The drawing under review shows one solid part. Ordinate dimensions are in mm from its lowest x, y, z. Round coordinates to 2 decimals unless told otherwise and drop trailing zeros. Order: outer loops, then holes, each group sorted by start corner. A loop starts at its lowest first (then second) coordinate and runs counter-clockwise, first axis right, second up.
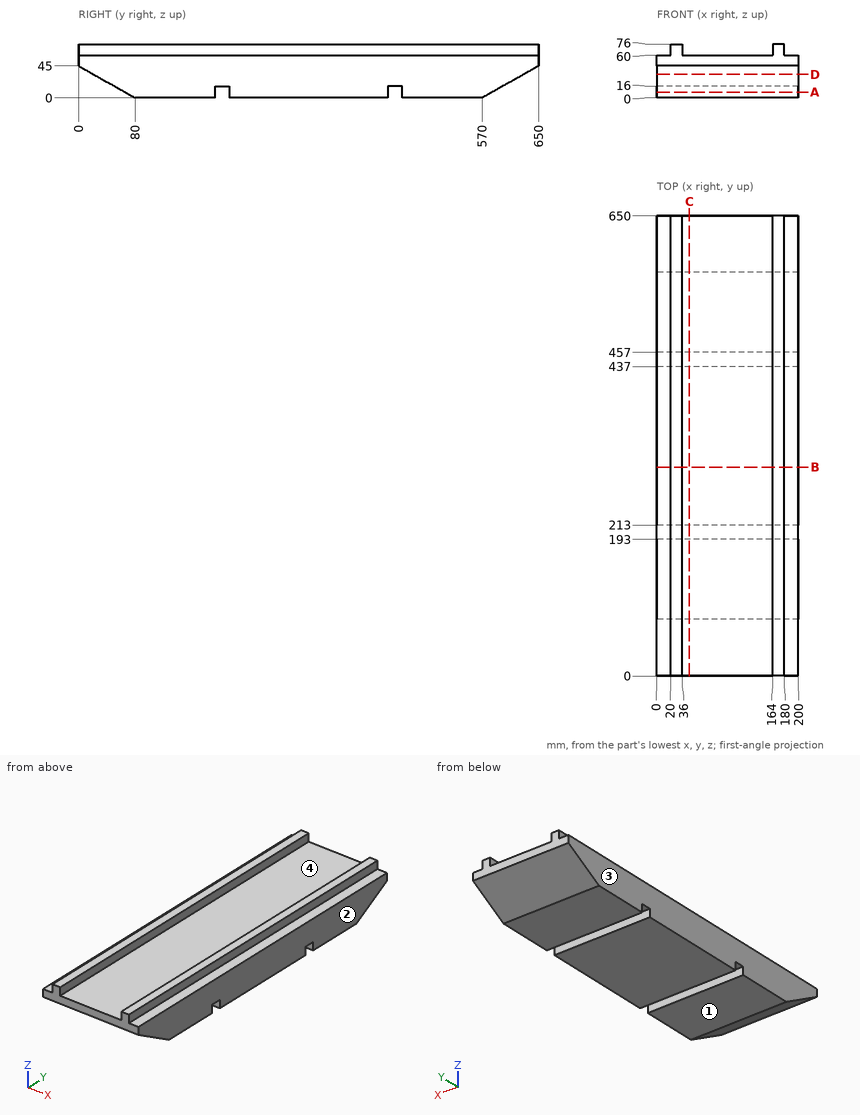
(1) To check wall thickness, follow L1, parallel to Z at x = 16.5, y = 365.5; L2, parallel to Y at x = 174, z = 11; L3, parallel to Y at x = 64, z = 12. State the ranges of each line that lie inside material, in increasing order.
(2) We need section C-C (x = 46). Give the boundary of the cut face in (y, z), and give its area (3 significant figures).
(3) The part is to be moulded in two halves that separate along X. For the marked faces 1, 2, 3 and 4, say which applies: pulls with the +X half, pulls with the -X half, needs draft (parallel to the pull), parting line crosses it, or undercut.
(4) Clearance check with flat-ended pins moving along their axes: P1, Ø13, axis at y = 423.5, z = 67.5, coming from the -X side; P2, Ø8, axis at x = 117, z = 10.5, coming from the +Y side; P3, Ø13, axis at y = 396.5, z = 70.5, coming from the +X side. State where each tip first meets the part, or that it passes through.
(5) We need section B-B (y = 295). Give the boundary of the cut face in (x, z), and give its area (3 significant figures).
(6) We need section A-A (z = 8). Give the boundary of the cut face in (x, y).
(7) We need section D-D (z = 33). Give the boundary of the cut face in (x, y).
Verdict:
1. L1: z = 0 to 60
1. L2: y = 60.44 to 193, 213 to 437, 457 to 589.56
1. L3: y = 58.67 to 193, 213 to 437, 457 to 591.33
2. outline: (0, 45) - (80, 0) - (193, 0) - (193, 16) - (213, 16) - (213, 0) - (437, 0) - (437, 16) - (457, 16) - (457, 0) - (570, 0) - (650, 45) - (650, 60) - (0, 60) - close
2. area: 34,800 mm2
3. face 1: needs draft
3. face 2: pulls with the +X half
3. face 3: pulls with the -X half
3. face 4: undercut
4. P1: stops at x = 20
4. P2: stops at y = 595.78
4. P3: stops at x = 180
5. outline: (0, 0) - (200, 0) - (200, 60) - (180, 60) - (180, 76) - (164, 76) - (164, 60) - (36, 60) - (36, 76) - (20, 76) - (20, 60) - (0, 60) - close
5. area: 12,500 mm2
6. outline: (0, 65.78) - (200, 65.78) - (200, 193) - (0, 193) - close; (0, 213) - (200, 213) - (200, 437) - (0, 437) - close; (0, 457) - (200, 457) - (200, 584.22) - (0, 584.22) - close
7. outline: (0, 21.33) - (200, 21.33) - (200, 628.67) - (0, 628.67) - close
